from build123d import *

# Parameters (mm, degrees)
F1_DEPTH = 9.525
F0_R     = 7.9375
F2_DEPTH = 25.4
F3_DEPTH = 31.75
F5_D     = 9.525
F5_DEPTH = 12.7
F5_TIP   = 2.8615986981


with BuildPart() as f1:
    # F0 (on Front) → F1 (new body)
    with BuildSketch(Plane.XZ):
        with BuildLine():
            ThreePointArc((-2.933616207, 15.6015871292), (10.135197771, 12.2185674751), (15.875, 0))
            ThreePointArc((15.875, 0), (9.0714869373, -13.0278067896), (-5.5075196531, -14.8890178411))
            Line((-5.5075196531, -14.8890178411), (28.575, -27.4963065702))
            Line((28.575, -27.4963065702), (60.325, 27.4963065702))
            Line((60.325, 27.4963065702), (-2.933616207, 15.6015871292))
        make_face()
    extrude(amount=F1_DEPTH)

    # F0 (on Front) → F2 (join)
    with BuildSketch(Plane.XZ):
        with BuildLine():
            ThreePointArc((-5.5075196531, -14.8890178411), (9.0714869373, -13.0278067896), (15.875, 0))
            ThreePointArc((15.875, 0), (10.135197771, 12.2185674751), (-2.933616207, 15.6015871292))
            ThreePointArc((-2.933616207, 15.6015871292), (-15.8187370392, 1.3353589349), (-5.5075196531, -14.8890178411))
        make_face()
        Circle(F0_R, mode=Mode.SUBTRACT)
    extrude(amount=F2_DEPTH)

    # F0 (on Front) → F3 (join)
    with BuildSketch(Plane.XZ):
        Polygon((71.3235226281, 21.1463065702), (60.325, 27.4963065702), (28.575, -27.4963065702), (39.5735226281, -33.8463065702), align=None)
    extrude(amount=F3_DEPTH)

    # F5
    with Locations(Plane(origin=(44.3360226281, 0, -25.5974145991), x_dir=(0, 1, 0), z_dir=(0.8660254038, 0, -0.5))):
        with Locations((-20.6375, 6.35), (-20.6375, 38.1)):
            Hole(F5_D / 2, depth=F5_DEPTH)
            with Locations((0, 0, -(F5_DEPTH + F5_TIP / 2))):  # 118° drill point
                Cone(0, F5_D / 2, F5_TIP, mode=Mode.SUBTRACT)


solid = f1.part
Geometry check sheet. Reference: the model listing, model coordinates, mm. A direction names the side the tool comes from. Give positions to 0.01 mm unless a question says otherwise; leave off trailing zeros. Use one line per item in the form item = value.
1) Sectioned sample at A-A (y = -11). Count the separate pieces of the cut face and the enclosed holes in it, and give its area (3 significant figures).
Working result:
separate_pieces = 2
enclosed_holes = 1
area = 1,400 mm^2
2) Depth check by flat-ended pin: pin 1 Ø10 at (x, z) = (36, 3.5) entering from -Y (3 decimals); pin 2 Ø2 at (y, z) = (-6, -16) entering from +X; pin 3 Ø10 at (x, y) = (-3.5, -9) entering from -Z; pin 4 Ø14.5 at (x, z) = (0, 0) entering from +Y. Enter the tip coordinate at first touch or a pass-through.
Working result:
pin_1 = -9.525
pin_2 = 50.45
pin_3 = -17.48
pin_4 = through
3) Draft check along Y on faces 1 (the face through (50, -31.75, -3)), 2 (the face through (56.9, -25.04, 9.04)), 3 (the face through (42.65, -25.18, -15.64)), 4 (the face through (34, -15.65, -30.63)). Enter one of: released by +Y, released by -Y, zero draft, split by the parting line, or undercut.
Working result:
face_1 = released by -Y
face_2 = undercut
face_3 = undercut
face_4 = zero draft
4) Material ranges on probe 1 along Z at (x, y) = (0, -11) (1 decimal); probe 2 along X at (y, z) = (-22, -3); probe 3 along Y at (x, z) = (17, -3.5) (3 decimals), recorded low to high. Write a range as from..to.
Working result:
probe_1 = -15.9..-7.9, 7.9..15.9
probe_2 = -15.59..-7.35, 7.35..15.59, 42.72..57.38
probe_3 = -9.525..0
5) Access from +Z, -Z, +X, -X, +Y, -Y to the whole of each face (thin tool, end or side, straight path). Record for faces 5 (the face through (44.67, -20.48, 0.38)), 6 (the face through (27, 0, -3)), 7 (the face through (-7.3, -25.4, 3.8)).
Working result:
face_5 = +Z, -Y
face_6 = +Z, -Z, +X, -X, +Y
face_7 = +Z, -Z, -X, -Y
